Source: CAD feature listing. Evaluate the final solid. Frame: model axes, mm. Face numbers are marked on the shaded views. A direction names the side the tool comes from. Coordinates: 2 decimals unless noted, no trailing zeros. Order: outer loops, then holes, each group sorted by start corner. A loop starts at its lowest first (then second) coordinate and runs counter-clockwise, first axis right, second up.
Item 1: Section B-B on y = -5.75. State how many separate pieces and enclosed holes the cut face has, then the cut area to 3 significant figures.
Item 2: Reachability of the marked faces 1, 2, 3 and 4 from +Z, -Z, +X, -X, +Y, -Y: full face, straight path, thin tool, end or side. Return the list, or none.
Item 3: Mould query, pull axis X, two halves, no side actions, for the marked faces 5, 6 and 7. Classes: released by +X, released by -X, zero draft, split by the parting line, or undercut.
Item 4: Section D-D on x = 28. Return the cut outline in (y, z), then the cut area to 3 significant figures.
Item 5: Ray query, line 1 (X direction, y = -6.25, z = 4); line 2 (X direction, y = -6.5, z = 45); line 3 (X direction, y = 7.25, z = -1.5). Return the intervals inside material, ascending.
Item 6: Contact query for flat-ended pins moving along their axis: P1, Ø1, axis at y = 1.5, z = -25, coming from the +X side; P2, Ø2, axis at x = -7, y = -9, coming from the +Z side; P3, Ø6, axis at x = 51.5, y = -0.5, coming from the -Z side. Output: stop coordinate, or through.
Item 7: Section C-C on x = -30.5. Return the cut outline in (y, z).
Item 8: Section A-A on z = 0. Return the cut outline in (x, y), then the cut area to 3 significant figures.
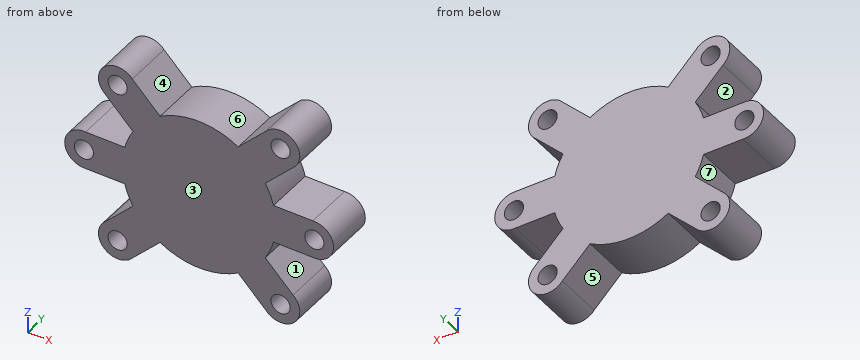
from build123d import *

# Parameters (mm, degrees)
F0_R     = 5
F0_R_2   = 30
F1_DEPTH = 12.7


with BuildPart() as f1:
    # F0 (on Front) → F1 (new body, symmetric)
    with BuildSketch(Plane.XZ):
        with BuildLine():
            Line((-48.8836239391, 34.7906785013), (-34.438939242, 20.3459938043))
            ThreePointArc((-34.438939242, 20.3459938043), (-36.9551813005, 15.3073372946), (-38.7387976639, 9.9652172859))
            Line((-38.7387976639, 9.9652172859), (-59.1666666667, 9.9652172859))
            ThreePointArc((-59.1666666667, 9.9652172859), (-70, 0), (-59.1666666667, -9.9652172859))
            Line((-59.1666666667, -9.9652172859), (-38.7387976639, -9.9652172859))
            ThreePointArc((-38.7387976639, -9.9652172859), (-36.9551813005, -15.3073372946), (-34.438939242, -20.3459938043))
            Line((-34.438939242, -20.3459938043), (-48.8836239391, -34.7906785013))
            ThreePointArc((-48.8836239391, -34.7906785013), (-49.4974746831, -49.4974746831), (-34.7906785013, -48.8836239391))
            Line((-34.7906785013, -48.8836239391), (-20.3459938043, -34.438939242))
            ThreePointArc((-20.3459938043, -34.438939242), (0, -40), (20.3459938043, -34.438939242))
            Line((20.3459938043, -34.438939242), (34.7906785013, -48.8836239391))
            ThreePointArc((34.7906785013, -48.8836239391), (49.4974746831, -49.4974746831), (48.8836239391, -34.7906785013))
            Line((48.8836239391, -34.7906785013), (34.438939242, -20.3459938043))
            ThreePointArc((34.438939242, -20.3459938043), (36.9551813005, -15.3073372946), (38.7387976639, -9.9652172859))
            Line((38.7387976639, -9.9652172859), (59.1666666667, -9.9652172859))
            ThreePointArc((59.1666666667, -9.9652172859), (70, 0), (59.1666666667, 9.9652172859))
            Line((59.1666666667, 9.9652172859), (38.7387976639, 9.9652172859))
            ThreePointArc((38.7387976639, 9.9652172859), (36.9551813005, 15.3073372946), (34.438939242, 20.3459938043))
            Line((34.438939242, 20.3459938043), (48.8836239391, 34.7906785013))
            ThreePointArc((48.8836239391, 34.7906785013), (49.4974746831, 49.4974746831), (34.7906785013, 48.8836239391))
            Line((34.7906785013, 48.8836239391), (20.3459938043, 34.438939242))
            ThreePointArc((20.3459938043, 34.438939242), (0, 40), (-20.3459938043, 34.438939242))
            Line((-20.3459938043, 34.438939242), (-34.7906785013, 48.8836239391))
            ThreePointArc((-34.7906785013, 48.8836239391), (-49.4974746831, 49.4974746831), (-48.8836239391, 34.7906785013))
        make_face()
        with Locations((-42.4264068712, -42.4264068712)):
            Circle(F0_R, mode=Mode.SUBTRACT)
        with Locations((42.4264068712, -42.4264068712)):
            Circle(F0_R, mode=Mode.SUBTRACT)
        with Locations((-60, 0)):
            Circle(F0_R, mode=Mode.SUBTRACT)
        with Locations((-42.4264068712, 42.4264068712)):
            Circle(F0_R, mode=Mode.SUBTRACT)
        Circle(F0_R_2, mode=Mode.SUBTRACT)
        with Locations((60, 0)):
            Circle(F0_R, mode=Mode.SUBTRACT)
        with Locations((42.4264068712, 42.4264068712)):
            Circle(F0_R, mode=Mode.SUBTRACT)
        Circle(F0_R_2)
    extrude(amount=F1_DEPTH, both=True)


solid = f1.part
Answer list:
1. separate pieces: 1
1. enclosed holes: 6
1. area: 7,940 mm2
2. face 1: +X, +Y, -Y
2. face 2: -X, +Y, -Y
2. face 3: +Z, -Z, +X, -X, -Y
2. face 4: +Z, +Y, -Y
3. face 5: undercut
3. face 6: undercut
3. face 7: released by -X
4. outline: (-12.7, -42.09) - (12.7, -42.09) - (12.7, 42.09) - (-12.7, 42.09) - close
4. area: 2,140 mm2
5. line 1: x = -69.17 to -63, -57 to 57, 63 to 69.17
5. line 2: x = -52.09 to -46.71, -38.14 to -30.91, 30.91 to 38.14, 46.71 to 52.09
5. line 3: x = -69.89 to -64.77, -55.23 to 55.23, 64.77 to 69.89
6. P1: stops at x = 39.59
6. P2: stops at z = 39.55
6. P3: stops at z = -50.37
7. outline: (-12.7, -44.59) - (12.7, -44.59) - (12.7, 44.59) - (-12.7, 44.59) - close
8. outline: (-70, -12.7) - (-65, -12.7) - (-65, 12.7) - (-70, 12.7) - close; (-55, -12.7) - (55, -12.7) - (55, 12.7) - (-55, 12.7) - close; (65, -12.7) - (70, -12.7) - (70, 12.7) - (65, 12.7) - close
8. area: 3,050 mm2
